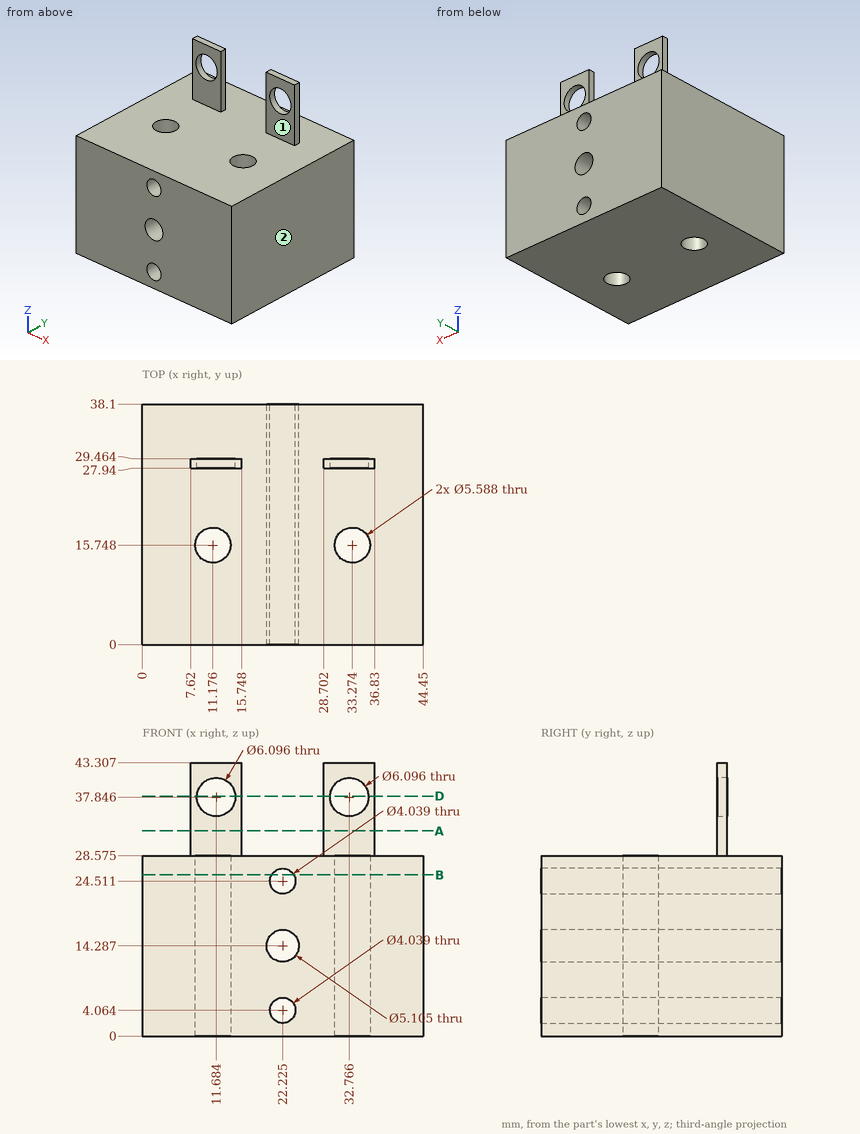
Print and shaded views of the part. All mm, measured from the part's lowest x, y and z. A direction names the side the tool comes from. Give positions to 0.01 mm unless a question says otherwise; leave off trailing zeros. Order: outer loops, then holes, each group sorted by start corner. A loop starts at its lowest first (then second) coordinate and runs counter-clockwise, first axis right, second up. Notation, with made-up numbers: (83, 1) - (118, 1) arc R26 cw to (118, 26) - close; hole circle Ø4 at (30, 77). An arc over 180 degrees is marked (long way). One line per item, written item: value.
Item 1: Slice it at A-A (z = 32.5). List the corners of the cut face in (x, y) (1 decimal).
Response values:
outline: (7.6, 27.9) - (15.7, 27.9) - (15.7, 29.5) - (7.6, 29.5) - close; (28.7, 27.9) - (36.8, 27.9) - (36.8, 29.5) - (28.7, 29.5) - close
Item 2: Tool access for the marked faces 1 and 2: list every direction of +Z, -Z, +X, -X, +Y, -Y with a clear straight run to the whole face (end or side of a thin tool).
Response values:
face 1: +Z, +X, -X, -Y
face 2: +Z, -Z, +X, +Y, -Y
Item 3: Wall check: line 1 (Z direction, x = 15, y = 32.5) (1 decimal); line 2 (Y direction, x = 14.5, z = 42) (1 decimal); line 3 (X direction, y = 27, z = 13). Give the ranges that are in metal, low to high.
Response values:
line 1: 0 to 28.6
line 2: 27.9 to 29.5
line 3: 0 to 20.02, 24.43 to 44.45
Item 4: Pin check, flat tips, straight feed: pin 1 Ø0.5 at (y, z) = (29, 37) entering from -X; pin 2 Ø10 at (x, z) = (11.684, 37.846) entering from +Y; pin 3 Ø9 at (x, z) = (34, 39.5) entering from -Y; pin 4 Ø8 at (x, z) = (35, 16) entering from -Y. Stop position of each tip, or through.
Response values:
pin 1: x = 7.62
pin 2: y = 29.46
pin 3: y = 27.94
pin 4: y = 0
Item 5: Slice it at D-D (z = 38). List the corners of the cut face in (x, y) (1 decimal).
Response values:
outline: (7.6, 27.9) - (8.6, 27.9) - (8.6, 29.5) - (7.6, 29.5) - close; (14.7, 27.9) - (15.7, 27.9) - (15.7, 29.5) - (14.7, 29.5) - close; (28.7, 27.9) - (29.7, 27.9) - (29.7, 29.5) - (28.7, 29.5) - close; (35.8, 27.9) - (36.8, 27.9) - (36.8, 29.5) - (35.8, 29.5) - close
Item 6: Slice it at B-B (z = 25.5). Give the number of separate pieces and of enclosed holes in the cut face, then the cut area to 3 significant figures.
Response values:
separate pieces: 2
enclosed holes: 2
area: 1,510 mm2
